Could you check a few things on this drawing? It's one solid part, dimensions in mm from its lowest x, y, z. A direction names the side the tool comes from. Round coordinates to 2 decimals unless told otherwise and drop trailing zeros. Loops run counter-clockwise (first coordinate to the right, second up) from the corner with the lowest first, then second, coordinate; pieces in that order, holes last. Notation, with made-up numbers: M -6.5,72.5 L 30.5,72.5 A12 ccw 30.5,87.5 Z; hole C 22.5,-35 d3. An arc over 180 degrees is marked long. Answer as a JSON object with one key per item and string values.
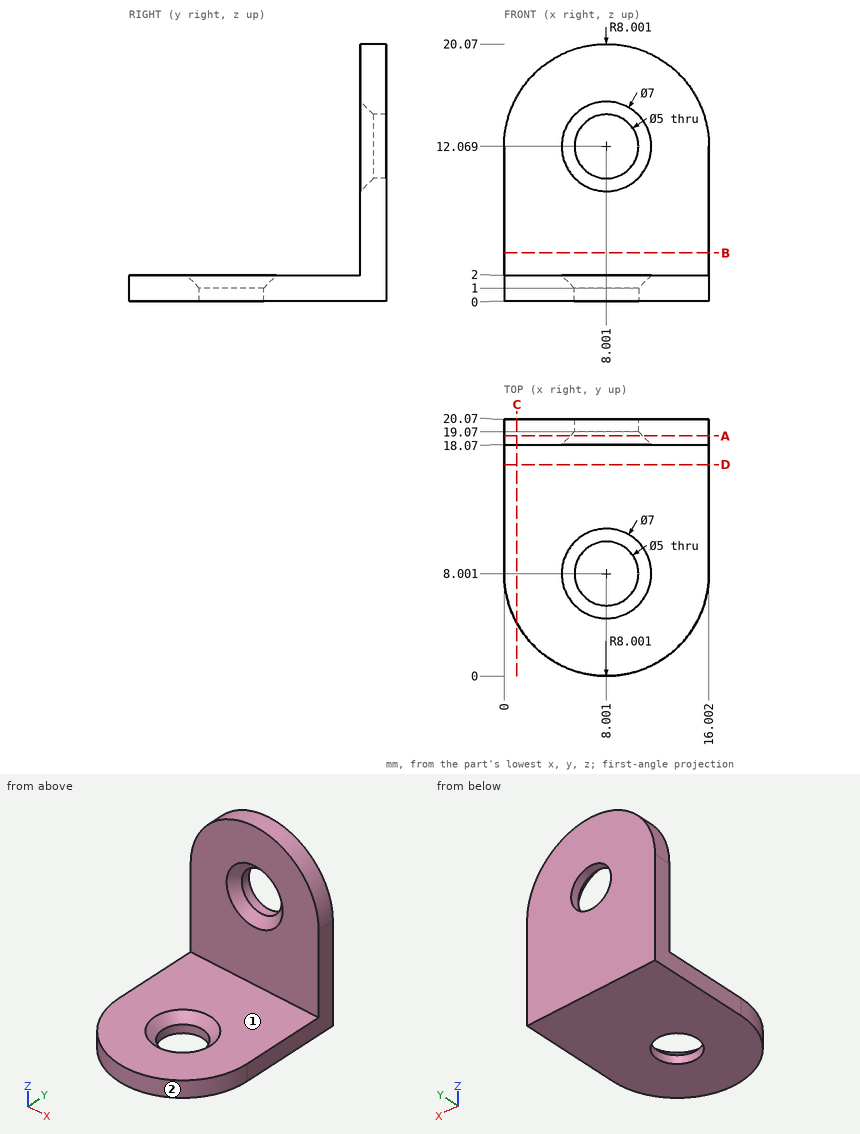
Item 1: I want a section at A-A, the plane y = 18.75. Please give me the cut outline in (x, z), then the cut area to 3 significant figures.
Resolved:
{"outline": "M 0,0 L 16,0 L 16,12.07 A8 ccw 0,12.07 Z; hole C 8,12.07 d5.64", "area": "269 mm²"}
Item 2: Please list where these lines run through material, in increasing order: probe 1 along Z at (x, y) = (7.25, 15); probe 2 along Y at (x, z) = (9.75, 3.5); probe 3 along Z at (x, y) = (10, 18.5). Write a range as from..to.
Resolved:
{"probe 1": "0..2", "probe 2": "18.07..20.07", "probe 3": "0..9.74, 14.4..19.82"}
Item 3: I want a section at D-D, the plane y = 16.5. Please give me the cut outline in (x, z).
Resolved:
{"outline": "M 0,0 L 16,0 L 16,2 L 0,2 Z"}
Item 4: I want a section at B-B, the plane z = 3.75. Please give me the cut outline in (x, y), then the cut area to 3 significant figures.
Resolved:
{"outline": "M 0,18.07 L 16,18.07 L 16,20.07 L 0,20.07 Z", "area": "32.0 mm²"}
Item 5: I'm going to push flat-ended pins straight in: pin 1 Ø6 at (x, y) = (7.5, 4.5) entering from +Z; pin 2 Ø5 at (x, y) = (8.5, 8) entering from +Z; pin 3 Ø5 at (x, z) = (11.5, 8) entering from -Y; pin 4 Ø3 at (x, y) = (13.5, 7) entering from -Z. Where does each tip first touch, or does it pass through?
Resolved:
{"pin 1": "z = 2", "pin 2": "z = 1.5", "pin 3": "y = 18.07", "pin 4": "z = 0"}
Item 6: On a 3-axis mill with a long thin cutter (end or side, diameter ignored), from which of +Z, -Z, +X, -X, +Y, -Y can I reach the whole of each face in a straight line? I mean the marked faces 1 and 2. Say none if no direction works.
Resolved:
{"face 1": "+Z, +X, -X, -Y", "face 2": "+Z, -Z, -Y"}
Item 7: I want a section at C-C, the plane x = 1. Please give me the cut outline in (y, z).
Resolved:
{"outline": "M 4.13,0 L 20.07,0 L 20.07,15.94 L 18.07,15.94 L 18.07,2 L 4.13,2 Z"}
